```python
from build123d import *

# Parameters (mm, degrees)
F0_W     = 28.3464
F0_H     = 31.1658
F1_DEPTH = 3.81
F2_W     = 22.5044
F2_H     = 28.4988
F3_DEPTH = 1.8288
F4_R     = 1.1303
F5_DEPTH = 28.3474
F6_R     = 3.2512
F6_W     = 20.4724
F6_H     = 10.16
F7_DEPTH = 3.811


with BuildPart() as f1:
    # F0 (on Top) → F1 (new body)
    with BuildSketch(Plane.XY):
        Rectangle(F0_W, F0_H)
    extrude(amount=F1_DEPTH)

    # F2 (on face) → F3 (cut)
    with BuildSketch(Plane.XY.offset(3.81)):
        Rectangle(F2_W, F2_H)
    extrude(amount=-F3_DEPTH, mode=Mode.SUBTRACT)

    # F4 (on face) → F5 (cut, through all)
    with BuildSketch(Plane(origin=(-14.1732, 0, 0), x_dir=(0, -1, 0), z_dir=(-1, 0, 0))):
        with Locations((9.2329, 2.2098)):
            Circle(F4_R)
        with Locations((-9.2329, 2.2098)):
            Circle(F4_R)
    extrude(amount=-F5_DEPTH, mode=Mode.SUBTRACT)

    # F6 (on face) → F7 (cut, through all)
    with BuildSketch(Plane(origin=(0, 0, 0), x_dir=(1, 0, 0), z_dir=(0, 0, -1))):
        with Locations((0, 8.0899)):
            Circle(F6_R)
        with Locations((0, -7.3279)):
            Rectangle(F6_W, F6_H)
    extrude(amount=-F7_DEPTH, mode=Mode.SUBTRACT)


solid = f1.part
```
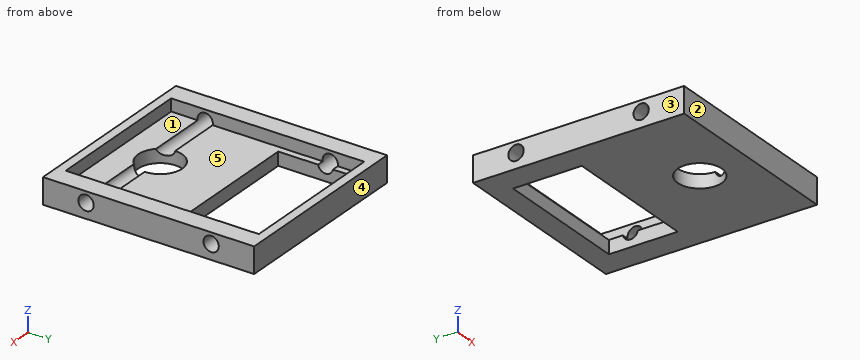
Read the model definition and answer for the solid it produces. Units are mm, in the model's axes. Face numbers are marked on the shaded views. A direction names the side the tool comes from. Coordinates: 2 decimals unless noted, no trailing zeros. Order: outer loops, then holes, each group sorted by start corner. A loop starts at its lowest first (then second) coordinate and runs counter-clockwise, first axis right, second up. Notation, with made-up numbers: (8, -3.5) - (17, -3.5) arc R13 ccw to (17, 14.5) - close; hole circle Ø10 at (11.5, 86). An arc over 180 degrees is marked (long way). Answer as a JSON object with one key per item and string values. Group by question number.
Item 1: Section C-C (x = 0) is taken. Give the vertices of the cut face in (y, z), plus the area to 3 significant figures.
Item 2: Section A-A (y = 4) is taken. Give the vertices of the cut face in (x, z), plus the area to 3 significant figures.
Item 3: The mould has two halves that part along X. Classify the marked faces 1, 2 and 3: +X half, -X half, draft (parallel to the pull), parting line (faces both ways), or undercut.
Item 4: A tool of negligible diameter and unlimited length cuts with its end or side. For the marked faces 4 and 5, from which of +Z, -Z, +X, -X, +Y, -Y can it reach the whole face along a straight path? Write none if from no direction.
Item 5: Section B-B (x = 5) is taken. Give the vertices of the cut face in (y, z), plus the area to 3 significant figures.
Item 6: A flat-ended cylindrical pin translates along its axis: P1, Ø6, axis at x = 5.5, y = 4, coming from the +Z side. Find the tip coordinate at first contact, or state that the pin passes through.
Item 7: Section D-D (y = 9.5) is taken. Give the vertices of the cut face in (x, z), plus the area to 3 significant figures.
Item 8: Consider probe 1 along Y at (x, z) = (0, 1.1); probe 2 along X at (y, z) = (3, 0.55); probe 3 along X at (y, z) = (11, 3.3). Determine where each line is inside the solid, lowest interval first. Write a range as from..to.
Results are:
{
 "1": {"outline": "(-15.58, 0) - (-11.34, 0) - (-11.34, 1.98) - (-14.25, 1.98) - (-14.25, 3.81) - (-15.58, 3.81) - close; (-4.84, 0) - (2.25, 0) - (2.25, 1.98) - (-4.84, 1.98) - close; (12.41, 0) - (15.58, 0) - (15.58, 3.81) - (14.25, 3.81) - (14.25, 1.98) - (12.41, 1.98) - close", "area": "33.6 mm^2"},
 "2": {"outline": "(-14.17, 0) - (-10.24, 0) - (-10.24, 1.98) - (-11.25, 1.98) - (-11.25, 3.81) - (-14.17, 3.81) - close; (10.24, 0) - (14.17, 0) - (14.17, 3.81) - (11.25, 3.81) - (11.25, 1.98) - (10.24, 1.98) - close", "area": "26.3 mm^2"},
 "3": {"face 1": "undercut", "face 2": "draft", "face 3": "-X half"},
 "4": {"face 4": "+Z, -Z, +X, -X, +Y", "face 5": "+Z"},
 "5": {"outline": "(-15.58, 0) - (2.25, 0) - (2.25, 1.98) - (-8.13, 1.98) arc R1.13 cw to (-10.34, 1.98) - (-14.25, 1.98) - (-14.25, 3.81) - (-15.58, 3.81) - close; (12.41, 0) - (15.58, 0) - (15.58, 3.81) - (14.25, 3.81) - (14.25, 1.98) - (12.41, 1.98) - close", "area": "45.0 mm^2"},
 "6": {"P1": "stops at z = 1.98"},
 "7": {"outline": "(-14.17, 0) - (-10.24, 0) - (-10.24, 1.11) - (-14.17, 1.11) - close; (-14.17, 3.31) - (-11.25, 3.31) - (-11.25, 3.81) - (-14.17, 3.81) - close; (10.24, 0) - (14.17, 0) - (14.17, 1.11) - (10.24, 1.11) - close; (11.25, 3.31) - (14.17, 3.31) - (14.17, 3.81) - (11.25, 3.81) - close", "area": "11.7 mm^2"},
 "8": {"probe 1": "y = -15.58..-11.34, -4.84..2.25, 12.41..15.58", "probe 2": "x = -14.17..-10.24, 10.24..14.17", "probe 3": "x = -14.17..-11.25, 11.25..14.17"}
}
